Geometry check sheet. Reference: drawing and pictorial views, mm from the part's lowest x, y, z. A direction names the side the tool comes from. Give positions to 0.01 mm unless a question says otherwise; leave off trailing zeros. Loops run counter-clockwise (first coordinate to the right, second up) from the corner with the lowest first, then second, coordinate; pieces in that order, holes last. Notation, with made-up numbers: (-18, 64.5) - (23, 64.5) arc R17 cw to (23, 88.5) - close; hole circle Ø1 at (54, 59.5). An arc over 180 degrees is marked (long way). One line per question, with ' | ' between items. Start each with the question number.
1. Section check B-B, the plane z = 12.5. Enter the section's corners in (x, y).
2. Section check C-C, the plane y = 2. Enter the section's corners in (x, z), then the cut area to 3 significant figures.
3. Thickness scan on line 1 along X through (y, z) = (2.4, 12.5); line 2 along Z through (x, y) = (26, 1.25); line 3 along Z through (x, y) = (8, 1.5). Record the ranges inside material, lowest first. Write a range as from..to.
4. Section check D-D, the plane y = 11. Enter the section's corners in (x, z), then the cut area to 3 significant figures.
5. Depth check by flat-ended pin: pin 1 Ø5.5 at (x, z) = (50, 52.5) entering from +Y; pin 2 Ø10 at (x, y) = (31, 16) entering from +Z. Enter the tip coordinate at first touch or a pass-through.
6. Section check A-A, the plane x = 45. Enter the section's corners in (y, z).
7. Tool access check on the marked faces 1 and 2. Record the directions out of +Z, -Z, +X, -X, +Y, -Y that give a thin tool (end or side, any length) a straight path to the whole face; none if there is none.
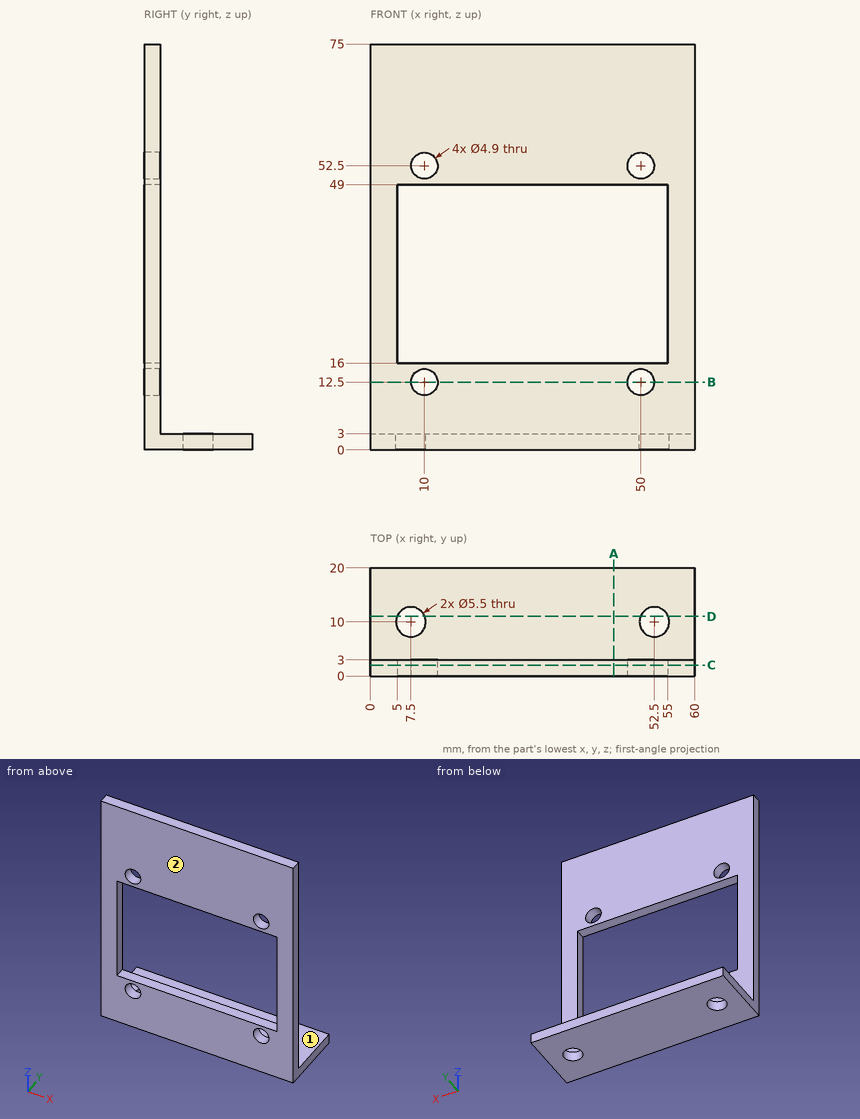
Results list:
1) outline: (0, 0) - (7.55, 0) - (7.55, 3) - (0, 3) - close; (12.45, 0) - (47.55, 0) - (47.55, 3) - (12.45, 3) - close; (52.45, 0) - (60, 0) - (60, 3) - (52.45, 3) - close
2) outline: (0, 0) - (60, 0) - (60, 75) - (0, 75) - close; hole (5, 16) - (55, 16) - (55, 49) - (5, 49) - close; hole circle Ø4.9 at (10, 12.5); hole circle Ø4.9 at (10, 52.5); hole circle Ø4.9 at (50, 12.5); hole circle Ø4.9 at (50, 52.5) | area: 2,770 mm²
3) line 1: 0..7.55, 12.45..47.55, 52.45..60 | line 2: 0..16, 49..75 | line 3: 0..11.08, 13.92..16, 49..51.08, 53.92..75
4) outline: (0, 0) - (4.94, 0) - (4.94, 3) - (0, 3) - close; (10.06, 0) - (49.94, 0) - (49.94, 3) - (10.06, 3) - close; (55.06, 0) - (60, 0) - (60, 3) - (55.06, 3) - close | area: 149 mm²
5) pin 1: y = 3 | pin 2: z = 3
6) outline: (0, 0) - (20, 0) - (20, 3) - (3, 3) - (3, 16) - (0, 16) - close; (0, 49) - (3, 49) - (3, 75) - (0, 75) - close
7) face 1: +Z, +X, -X, +Y | face 2: +Z, -Z, +X, -X, -Y
